```python
from build123d import *

# Parameters (mm, degrees)
BOSS_EXTRUDE1_DEPTH = 1.5
SKETCH2_R           = 2.75
BOSS_EXTRUDE2_DEPTH = 6
SKETCH3_W           = 1.1
SKETCH3_H           = 1.45
SKETCH3_W_2         = 1.45
SKETCH3_H_2         = 1.1
CUT_EXTRUDE1_DEPTH  = 6
CHAMFER1_SIZE       = 0.3
FILLET1_R           = 1
SKETCH4_R           = 1.25
BOSS_EXTRUDE3_DEPTH = 0.01
DOME2_FACE_RADIUS   = 1.25
DOME2_HEIGHT        = 1.25
DOME3_FACE_RADIUS   = 1.25
DOME3_HEIGHT        = 1.25
FILLET3_R           = 0.2


with BuildPart() as part:
    # Sketch1 → Boss-Extrude1 (new body)
    with BuildSketch(Plane(origin=(0, 0, 0), x_dir=(1, 0, 0), z_dir=(0, 1, 0))):
        with BuildLine():
            Line((-7.324675649, 4.396717546), (4.675324351, 4.396717546))
            ThreePointArc((4.675324351, 4.396717546), (5.382431132, 4.103824327), (5.675324351, 3.396717546))
            Line((5.675324351, 3.396717546), (5.675324351, -8.603282454))
            ThreePointArc((5.675324351, -8.603282454), (5.382431132, -9.310389235), (4.675324351, -9.603282454))
            Line((4.675324351, -9.603282454), (-7.324675649, -9.603282454))
            ThreePointArc((-7.324675649, -9.603282454), (-8.03178243, -9.310389235), (-8.324675649, -8.603282454))
            Line((-8.324675649, -8.603282454), (-8.324675649, 3.396717546))
            ThreePointArc((-8.324675649, 3.396717546), (-8.03178243, 4.103824327), (-7.324675649, 4.396717546))
        make_face()
    extrude(amount=BOSS_EXTRUDE1_DEPTH)

    # Sketch2 → Boss-Extrude2 (add)
    with BuildSketch(Plane.XZ):
        with Locations(Location((-1.324675649, 2.603282454, 0), (0, 0, 270))):
            Circle(SKETCH2_R)
    extrude(amount=BOSS_EXTRUDE2_DEPTH)

    # Sketch3 → Cut-Extrude1 (cut)
    with BuildSketch(Plane.XZ.offset(6)):
        with Locations((-1.324675649, 3.878282454)):
            Rectangle(SKETCH3_W, SKETCH3_H)
        with Locations((-0.049675649, 2.603282454)):
            Rectangle(SKETCH3_W_2, SKETCH3_H_2)
        with Locations((-1.324675649, 2.603282454)):
            Rectangle(SKETCH3_W, SKETCH3_H_2)
        with Locations((-2.599675649, 2.603282454)):
            Rectangle(SKETCH3_W_2, SKETCH3_H_2)
        with Locations((-1.324675649, 1.328282454)):
            Rectangle(SKETCH3_W, SKETCH3_H)
    extrude(amount=-CUT_EXTRUDE1_DEPTH, mode=Mode.SUBTRACT)

    # Chamfer1
    chamfer1_edges = [part.edges().sort_by_distance(p)[0] for p in [
        (-0.774675649, -6, 3.878282454),
        (-0.049675649, -6, 3.153282454),
        (0.675324351, -6, 2.603282454),
        (-0.774675649, -6, 1.328282454),
        (-2.599675649, -6, 3.153282454),
        (-1.324675649, -6, 4.603282454),
        (-1.874675649, -6, 3.878282454),
        (-3.324675649, -6, 2.603282454),
        (-2.599675649, -6, 2.053282454),
        (-1.874675649, -6, 1.328282454),
        (-1.324675649, -6, 0.603282454),
        (-0.049675649, -6, 2.053282454),
    ]]
    chamfer(chamfer1_edges, length=CHAMFER1_SIZE)

    # Fillet1
    fillet1_edges = [part.edges().sort_by_distance(p)[0] for p in [
        (-1.324675649, 0, 5.353282454),
    ]]
    fillet(fillet1_edges, radius=FILLET1_R)

    # Sketch4 → Boss-Extrude3 (add)
    with BuildSketch(Plane(origin=(0, 1.5, 0), x_dir=(1, 0, 0), z_dir=(0, 1, 0))):
        with Locations(Location((-3.324675649, -2.603282454, 0), (0, 0, 90))):
            Circle(SKETCH4_R)
        with Locations(Location((0.675324351, 1.396717546, 0), (0, 0, 90))):
            Circle(SKETCH4_R)
    extrude(amount=BOSS_EXTRUDE3_DEPTH)

    # Dome2: a dome of height H over a round flat face of radius A is a cap of a sphere of radius (A * A + H * H) / (2 * H)
    dome2_r = (DOME2_FACE_RADIUS * DOME2_FACE_RADIUS + DOME2_HEIGHT * DOME2_HEIGHT) / (2 * DOME2_HEIGHT)
    dome2_base = Plane((0.675324351, 1.51, -1.396717546), z_dir=(0, 1, 0))
    with Locations(dome2_base.offset(DOME2_HEIGHT - dome2_r)):
        dome2_ball = Sphere(dome2_r, mode=Mode.PRIVATE)
    add(split(dome2_ball, bisect_by=dome2_base, keep=Keep.TOP, mode=Mode.PRIVATE))

    # Dome3: a dome of height H over a round flat face of radius A is a cap of a sphere of radius (A * A + H * H) / (2 * H)
    dome3_r = (DOME3_FACE_RADIUS * DOME3_FACE_RADIUS + DOME3_HEIGHT * DOME3_HEIGHT) / (2 * DOME3_HEIGHT)
    dome3_base = Plane((-3.324675649, 1.51, 2.603282454), z_dir=(0, 1, 0))
    with Locations(dome3_base.offset(DOME3_HEIGHT - dome3_r)):
        dome3_ball = Sphere(dome3_r, mode=Mode.PRIVATE)
    add(split(dome3_ball, bisect_by=dome3_base, keep=Keep.TOP, mode=Mode.PRIVATE))

    # Fillet3
    fillet3_edges = [part.edges().sort_by_distance(p)[0] for p in [
        (5.382431132, 1.5, 9.310389235),
        (-1.324675649, 0, 9.603282454),
        (-8.03178243, 0, 9.310389235),
        (5.675324351, 1.5, 2.603282454),
        (5.382431132, 1.5, -4.103824327),
        (-1.324675649, 1.5, -4.396717546),
        (-8.03178243, 1.5, -4.103824327),
        (-8.324675649, 1.5, 2.603282454),
        (-8.03178243, 1.5, 9.310389235),
        (-1.324675649, 1.5, 9.603282454),
        (-8.324675649, 0, 2.603282454),
        (-8.03178243, 0, -4.103824327),
        (-1.324675649, 0, -4.396717546),
        (5.382431132, 0, -4.103824327),
        (5.675324351, 0, 2.603282454),
        (5.382431132, 0, 9.310389235),
    ]]
    fillet(fillet3_edges, radius=FILLET3_R)


solid = part.part
```
Verification items for the finished model (mm, model axes). A direction names the side the tool comes from. Coordinates: 2 decimals unless noted, no trailing zeros. Loops run counter-clockwise (first coordinate to the right, second up) from the corner with the lowest first, then second, coordinate; pieces in that order, holes last. Notation, with made-up numbers: (24.25, 65) -> (62.25, 65) arc R18 ccw to (62.25, 97) -> close; hole circle Ø10 at (-4, 25.25). An arc over 180 degrees is marked (long way). Put each result on its own line as item: value.
1. Thickness scan on line 1 (X direction, y = -5.5, z = 2.5); line 2 (Y direction, x = -7.5, z = 8.25); line 3 (X direction, y = -1.5, z = 0.75). Record the ranges inside material, lowest first.
Result set:
line 1: x = -4.07 to -3.32, 0.68 to 1.42
line 2: y = 0 to 1.5
line 3: x = -3.36 to -1.87, -0.77 to 0.71
2. Section check B-B, the plane z = 6.75. Record the boundary of the cut face in (x, y).
Result set:
outline: (-8.32, 0.2) arc R0.2 ccw to (-8.12, 0) -> (5.48, 0) arc R0.2 ccw to (5.68, 0.2) -> (5.68, 1.3) arc R0.2 ccw to (5.48, 1.5) -> (-8.12, 1.5) arc R0.2 ccw to (-8.32, 1.3) -> close
3. Section check A-A, the plane y = -0.5. Record the boundary of the cut face in (x, z), then the cut area to 3 significant figures.
Result set:
outline: circle Ø5.77 at (-1.32, 2.6); hole (-3.32, 2.05) -> (-1.87, 2.05) -> (-1.87, 0.6) -> (-0.77, 0.6) -> (-0.77, 2.05) -> (0.68, 2.05) -> (0.68, 3.15) -> (-0.77, 3.15) -> (-0.77, 4.6) -> (-1.87, 4.6) -> (-1.87, 3.15) -> (-3.32, 3.15) -> close
area: 18.5 mm^2
4. Section check C-C, the plane x = 4.5. Record the boundary of the cut face in (y, z), then the cut area to 3 significant figures.
Result set:
outline: (0, -4.2) arc R0.2 ccw to (0.2, -4.4) -> (1.3, -4.4) arc R0.2 ccw to (1.5, -4.2) -> (1.5, 9.4) arc R0.2 ccw to (1.3, 9.6) -> (0.2, 9.6) arc R0.2 ccw to (0, 9.4) -> close
area: 21.0 mm^2
5. Tool access check on faces 1 (the face through (-1, 1.5, 3)), 2 (the face through (5.675, 1, 3)), 3 (the face through (0, -3, 3.153)). Record the directions out of +Z, -Z, +X, -X, +Y, -Y that give a thin tool (end or side, any length) a straight path to the whole face; none if there is none.
Result set:
face 1: +Y
face 2: +Z, -Z, +X, +Y, -Y
face 3: -Y
6. Mould release check, pull along Z, two halves, no side actions. Record for faces 4 (the face through (-3, -6, 1)), 5 (the face through (-1.875, -3, 4)), 6 (the face through (-8.04, 0.742, -4.096)): pulls with the +Z half, pulls with the -Z half, needs draft (parallel to the pull), parting line crosses it, or undercut.
Result set:
face 4: needs draft
face 5: undercut
face 6: pulls with the -Z half
7. Gauge pin test, flat ends, axial feed: P1, Ø0.7, axis at y = -2, z = 1.5, coming from the +X side; P2, Ø4, axis at x = 0.5, z = 4.5, coming from the +Y side; P3, Ø0.7, axis at x = -3, y = -2, coming from the +Z side. Record the tip position at first contact, or that the pin passes through.
Result set:
P1: stops at x = 1.32
P2: stops at y = 1.5
P3: stops at z = 5.01
8. Section check D-D, the plane y = 2.25. Record the boundary of the cut face in (x, z), then the cut area to 3 significant figures.
Result set:
outline: circle Ø2.01 at (-3.32, 2.6); circle Ø2.01 at (0.68, -1.4)
area: 6.38 mm^2
